Part model, mm, in its own coordinate system. A direction names the side the tool comes from. Round coordinates to 2 decimals unless told otherwise and drop trailing zeros. Loops run counter-clockwise (first coordinate to the right, second up) from the corner with the lowest first, then second, coordinate; pieces in that order, holes last.
from build123d import *

# Parameters (mm, degrees)
F0_R          = 11
F0_R_2        = 8
F1_DEPTH      = 15
F1_DEPTH_BACK = 15
F4_R          = 3
F4_R_2        = 2
F5_DEPTH      = 10
F6_D          = 4
F6_DEPTH      = 18.0010001


with BuildPart() as f1:
    # F0 (on Top) → F1 (new body, two sides)
    with BuildSketch(Plane.XY) as f1_sk:
        Circle(F0_R)
        Circle(F0_R_2, mode=Mode.SUBTRACT)
    extrude(amount=F1_DEPTH)
    extrude(f1_sk.sketch, amount=-F1_DEPTH_BACK)

    # F4 (on offset) → F5 (join)
    with BuildSketch(Plane.YZ.offset(8)):
        Circle(F4_R)
        Circle(F4_R_2, mode=Mode.SUBTRACT)
    extrude(amount=F5_DEPTH)

    # F6 (through all, one way)
    with BuildSketch(Plane(origin=(0, 0, 0), x_dir=(0, 1, 0), z_dir=(-1, 0, 0))):
        with Locations((0, 0)):
            Circle(F6_D / 2)
    extrude(amount=-F6_DEPTH, mode=Mode.SUBTRACT)


solid = f1.part
1) Slice it at D-D, the plane x = 11.5. Give the cut face in (y, z), then the cut area to 3 significant figures.
Values:
outline: circle Ø6 at (0, 0); hole circle Ø4 at (0, 0)
area: 15.7 mm2
2) Slice it at B-B, the plane y = 0. Give the cut face in (x, z).
Values:
outline: (-11, -15) - (-8, -15) - (-8, 15) - (-11, 15) - close; (8, -15) - (11, -15) - (11, -3) - (18, -3) - (18, -2) - (8, -2) - close; (8, 2) - (18, 2) - (18, 3) - (11, 3) - (11, 15) - (8, 15) - close
3) Tool access for faces 4 (the face through (14.24, 2.86, 0.9)), 5 (the face through (18, 1, -2)): list every direction of +Z, -Z, +X, -X, +Y, -Y with a clear straight run to the whole face (end or side of a thin tool).
Values:
face 4: +X
face 5: +Z, -Z, +X, +Y, -Y
4) Slice it at C-C, the plane z = 0. Give the cut face in (x, y), then the cut area to 3 significant figures.
Values:
outline: (7.75, -2) arc R8 cw (long way) to (7.75, 2) - (18, 2) - (18, 3) - (10.58, 3) arc R11 ccw (long way) to (10.58, -3) - (18, -3) - (18, -2) - close
area: 182 mm2
5) Mould opens along Y. For faces 1 (the face through (-1.73, -7.81, -0.21)), 2 (the face through (-2, -8, -15)), 3 (the face through (-2.38, -10.74, 0.21)) say: released by +Y, released by -Y, zero draft, split by the parting line, or undercut.
Values:
face 1: undercut
face 2: zero draft
face 3: split by the parting line
6) Wall check: line 1 along Y through (x, z) = (15.75, 0); line 2 along Y through (x, z) = (0, -2); line 3 along X through (y, z) = (-4.5, -11.5). Give the ranges that are in metal, low to high.
Values:
line 1: y = -3 to -2, 2 to 3
line 2: y = -11 to -8, 8 to 11
line 3: x = -10.04 to -6.61, 6.61 to 10.04
7) Slice it at A-A, the plane x = 0. Give the cut face in (y, z).
Values:
outline: (-11, -15) - (-8, -15) - (-8, 15) - (-11, 15) - close; (8, -15) - (11, -15) - (11, 15) - (8, 15) - close
8) Drop flat-ended pins along their axis: pin 1 Ø10 at (y, z) = (8, 1.5) entering from -X; pin 2 Ø6 at (y, z) = (-5.5, 12) entering from -X; pin 3 Ø4 at (y, z) = (-3.5, 11.5) entering from +X. Give the stop position or say it passes through.
Values:
pin 1: stops at x = -10.58
pin 2: stops at x = -10.71
pin 3: stops at x = 10.9
